Verification items for the finished model (mm, model axes). Round coordinates to 2 decimals unless told otherwise and drop trailing zeros. Write each loop counter-clockwise with the first axis right and the second up, starting at its lowest first coordinate (ties: lowest second). Pieces come first, ordered by that corner, then holes. Notation, with made-up numbers: (10.5, -7.5) - (26.5, -7.5) arc R8 cw to (26.5, 6.5) - close; hole circle Ø3 at (40, 35.5). An arc over 180 degrees is marked (long way). Answer as a JSON object with one key per item and string values.
```python
from build123d import *

# Parameters (mm, degrees)
F1_DEPTH = 6.35


with BuildPart() as f1:
    # F0 (on Front) → F1 (new body)
    with BuildSketch(Plane.XZ):
        with BuildLine():
            Line((15.443564, 4.712719), (-40.843564, 4.712719))
            Line((-40.843564, 4.712719), (-40.843564, 0))
            Line((-40.843564, 0), (-15.885977, -4.712719))
            Line((-15.885977, -4.712719), (40.843564, -4.712719))
            Line((40.843564, -4.712719), (40.843564, 4.712719))
            Line((40.843564, 4.712719), (21.793564, 4.712719))
            ThreePointArc((21.793564, 4.712719), (18.618564, 1.537719), (15.443564, 4.712719))
        make_face()
    extrude(amount=F1_DEPTH)


solid = f1.part
```
Q1. Section check C-C, the plane z = -2.5. Record the cut outline in (x, y), then the cut area to 3 significant figures.
Geometry check:
{"outline": "(-27.6, -6.35) - (40.84, -6.35) - (40.84, 0) - (-27.6, 0) - close", "area": "435 mm2"}
Q2. Material ranges on line 1 along X through (y, z) = (-3.5, 3.25); line 2 along X through (y, z) = (-4.25, 4), recorded low to high. Write a range as [from, to].
Geometry check:
{"line 1": "x = [-40.84, 15.8], [21.44, 40.84]", "line 2": "x = [-40.84, 15.52], [21.71, 40.84]"}
Q3. Section check A-A, the plane z = 2.75. Record the cut outline in (x, y), then the cut area to 3 significant figures.
Geometry check:
{"outline": "(-40.84, -6.35) - (16.12, -6.35) - (16.12, 0) - (-40.84, 0) - close; (21.11, -6.35) - (40.84, -6.35) - (40.84, 0) - (21.11, 0) - close", "area": "487 mm2"}
Q4. Section check D-D, the plane x = -29. Record the cut outline in (y, z).
Geometry check:
{"outline": "(-6.35, -2.24) - (0, -2.24) - (0, 4.71) - (-6.35, 4.71) - close"}
Q5. Section check B-B, the plane y = -3. Record the cut outline in (x, z) (3 decimals).
Geometry check:
{"outline": "(-40.844, 0) - (-15.886, -4.713) - (40.844, -4.713) - (40.844, 4.713) - (21.794, 4.713) arc R3.175 cw to (15.444, 4.713) - (-40.844, 4.713) - close"}
